For this review, take the finished solid that the model builds, in its own axes (mm). A direction names the side the tool comes from. Give positions to 0.01 mm unless a question says otherwise; leave off trailing zeros. Write each loop counter-clockwise with the first axis right and the second up, starting at its lowest first coordinate (ties: lowest second). Pieces come first, ordered by that corner, then holes. Notation, with made-up numbers: (75.25, -20) -> (87.25, -20) arc R13 cw to (87.25, -6) -> close; hole circle Ø3 at (86.25, 15.25). An arc over 180 degrees is marked (long way). Write item = value, one per line.
```python
from build123d import *

# Parameters (mm, degrees)
SKETCH2_R           = 30
BOSS_EXTRUDE1_DEPTH = 10
SKETCH3_R           = 30
BOSS_EXTRUDE2_DEPTH = 20
SKETCH5_W           = 160
SKETCH5_H           = 60
BOSS_EXTRUDE3_DEPTH = 10


with BuildPart() as part:
    # Sketch2 → Boss-Extrude1 (new body)
    with BuildSketch(Plane.XY):
        with BuildLine():
            Line((0, -40), (-160, -40))
            ThreePointArc((-160, -40), (-200, 0), (-160, 40))
            Line((-160, 40), (0, 40))
            ThreePointArc((0, 40), (40, 0), (0, -40))
        make_face()
        Circle(SKETCH2_R, mode=Mode.SUBTRACT)
    boss_extrude1 = extrude(amount=BOSS_EXTRUDE1_DEPTH)

    # Sketch3 → Boss-Extrude2 (add)
    with BuildSketch(Plane.XY.offset(10)):
        with Locations((-160, 0)):
            Circle(SKETCH3_R)
    boss_extrude2 = extrude(amount=BOSS_EXTRUDE2_DEPTH)

    # Sketch5 → Boss-Extrude3 (add)
    with BuildSketch(Plane.XZ.offset(40)):
        with Locations((-80, -30)):
            Rectangle(SKETCH5_W, SKETCH5_H)
    extrude(amount=-BOSS_EXTRUDE3_DEPTH)

    # Mirror1: Boss-Extrude1, Boss-Extrude2 across plane
    add(boss_extrude1.mirror(Plane(origin=(0, 0, -25), x_dir=(1, 0, 0), z_dir=(0, 0, -1))))
    add(boss_extrude2.mirror(Plane(origin=(0, 0, -25), x_dir=(1, 0, 0), z_dir=(0, 0, -1))))


solid = part.part
```
(1) Take a section at D-D (z = 21). Write out the cut boundary in (x, y).
Answers below:
outline = circle Ø60 at (-160, 0)
(2) To check wall thickness, follow probe 1 along Z at (x, y) = (-36.5, -5.5); probe 2 along Z at (x, y) = (-170.5, -17); probe 3 along X at (y, z) = (0, 6). State the ranges of each line that lie inside material, in increasing order.
Answers below:
probe_1 = -60 to -50, 0 to 10
probe_2 = -80 to -50, 0 to 30
probe_3 = -200 to -30, 30 to 40
(3) Take a section at C-C (x = -59.5). Write out the cut boundary in (y, z).
Answers below:
outline = (-40, -60) -> (40, -60) -> (40, -50) -> (-30, -50) -> (-30, 0) -> (40, 0) -> (40, 10) -> (-40, 10) -> close
(4) Take a section at A-A (y = -20.5). Write out the cut boundary in (x, z).
Answers below:
outline = (-194.35, -60) -> (-181.9, -60) -> (-181.9, -80) -> (-138.1, -80) -> (-138.1, -60) -> (-21.9, -60) -> (-21.9, -50) -> (-194.35, -50) -> close; (-194.35, 0) -> (-21.9, 0) -> (-21.9, 10) -> (-138.1, 10) -> (-138.1, 30) -> (-181.9, 30) -> (-181.9, 10) -> (-194.35, 10) -> close; (21.9, -60) -> (34.35, -60) -> (34.35, -50) -> (21.9, -50) -> close; (21.9, 0) -> (34.35, 0) -> (34.35, 10) -> (21.9, 10) -> close
(5) For pin 1 (10 mm diameter, centred on x = -104.5, y = 17.5, fed in from +Z); pin 2 (5 mm diameter, centred on x = -174.5, z = 10.5, fed in from -Y); pin 3 (2 mm diameter, centred on y = -6, z = 12, fed in from -X), all flat-tipped, find the tip position at first contact; note any pin that passes through.
Answers below:
pin_1 = 10
pin_2 = -38.14
pin_3 = -189.58
(6) Take a section at B-B (y = 34). Write out the cut boundary in (x, z), plus the area to 3 significant figures.
Answers below:
outline = (-181.07, -60) -> (21.07, -60) -> (21.07, -50) -> (-181.07, -50) -> close; (-181.07, 0) -> (21.07, 0) -> (21.07, 10) -> (-181.07, 10) -> close
area = 4,040 mm^2
(7) Tool access review of faces 1 (the face through (-81, -30, -25)), 2 (the face through (-81, -40, -25)), 3 (the face through (-131.385, 9.011, -69.86)), 4 (the face through (0, -35, -25)), 5 (the face through (-131.385, 9.011, 19.86)): name each direction out of +Z, -Z, +X, -X, +Y, -Y from which nothing blocks a thin tool from reaching the whole face with its end or side.
Answers below:
face_1 = +X, -X, +Y
face_2 = +Z, -Z, +X, -X, -Y
face_3 = -Z
face_4 = +X, +Y, -Y
face_5 = +Z
(8) The part is to be moulded in two halves that separate along X. For faces 6 (the face through (-78, 1, 10)), 7 (the face through (-160, -35, -25)), 8 (the face through (-29.97, 1.32, 4.93)), 9 (the face through (39.99, 0.88, 4.93)), say which applies: released by +X, released by -X, zero draft, split by the parting line, or undercut.
Answers below:
face_6 = zero draft
face_7 = released by -X
face_8 = undercut
face_9 = released by +X
